```python
from build123d import *

# Parameters (mm, degrees)
BOSS_EXTRUDE1_DEPTH = 7.5
CUT_EXTRUDE3_DEPTH  = 5
SKETCH3_R           = 1.825
CUT_EXTRUDE4_DEPTH  = 13.5
SKETCH4_W           = 33.2
SKETCH4_H           = 26
CUT_EXTRUDE5_DEPTH  = 1
SKETCH5_W           = 2.5
SKETCH5_H           = 8
CUT_EXTRUDE6_DEPTH  = 5
BOSS_EXTRUDE2_DEPTH = 1
CUT_EXTRUDE8_DEPTH  = 10
SKETCH9_W           = 0.917517868
SKETCH9_H           = 1.289779541
SKETCH9_W_2         = 0.704402717
CUT_EXTRUDE9_DEPTH  = 1
CHAMFER1_SIZE       = 1
FILLET1_R           = 3.65


with BuildPart() as part:
    # Sketch1 → Boss-Extrude1 (new body)
    with BuildSketch(Plane(origin=(0, 0, 0), x_dir=(1, 0, 0), z_dir=(0, 1, 0))):
        with BuildLine():
            Line((-17.1, -15.5), (17.1, -15.5))
            ThreePointArc((17.1, -15.5), (18.514213562, -14.914213562), (19.1, -13.5))
            Line((19.1, -13.5), (19.1, 13.5))
            ThreePointArc((19.1, 13.5), (18.514213562, 14.914213562), (17.1, 15.5))
            Line((17.1, 15.5), (-17.1, 15.5))
            ThreePointArc((-17.1, 15.5), (-18.514213562, 14.914213562), (-19.1, 13.5))
            Line((-19.1, 13.5), (-19.1, -13.5))
            ThreePointArc((-19.1, -13.5), (-18.514213562, -14.914213562), (-17.1, -15.5))
        make_face()
    extrude(amount=BOSS_EXTRUDE1_DEPTH)

    # Sketch2 → Cut-Extrude3 (cut)
    with BuildSketch(Plane(origin=(0, 7.5, 0), x_dir=(1, 0, 0), z_dir=(0, 1, 0))):
        Polygon((-16.6, 5.5), (-9.1, 5.5), (-9.1, 13), (9.1, 13), (9.1, 5.5), (16.6, 5.5), (16.6, -5.5), (9.1, -5.5), (9.1, -13), (-9.1, -13), (-9.1, -5.5), (-16.6, -5.5), align=None)
    extrude(amount=-CUT_EXTRUDE3_DEPTH, mode=Mode.SUBTRACT)

    # Sketch3 → Cut-Extrude4 (cut)
    with BuildSketch(Plane(origin=(0, 7.5, 0), x_dir=(1, 0, 0), z_dir=(0, 1, 0))):
        with Locations((-12.425, 8.675)):
            Circle(SKETCH3_R)
        with Locations((12.425, 8.675)):
            Circle(SKETCH3_R)
        with Locations((12.425, -8.675)):
            Circle(SKETCH3_R)
        with Locations((-12.425, -8.675)):
            Circle(SKETCH3_R)
    extrude(amount=-CUT_EXTRUDE4_DEPTH, mode=Mode.SUBTRACT)

    # Sketch4 → Cut-Extrude5 (cut)
    with BuildSketch(Plane(origin=(0, 7.5, 0), x_dir=(1, 0, 0), z_dir=(0, 1, 0))):
        Rectangle(SKETCH4_W, SKETCH4_H)
    extrude(amount=-CUT_EXTRUDE5_DEPTH, mode=Mode.SUBTRACT)

    # Sketch5 → Cut-Extrude6 (cut)
    with BuildSketch(Plane(origin=(0, 7.5, 0), x_dir=(1, 0, 0), z_dir=(0, 1, 0))):
        with Locations((-17.85, 1.5)):
            Rectangle(SKETCH5_W, SKETCH5_H)
        with Locations((17.85, 1.5)):
            Rectangle(SKETCH5_W, SKETCH5_H)
    extrude(amount=-CUT_EXTRUDE6_DEPTH, mode=Mode.SUBTRACT)

    # Sketch6 → Boss-Extrude2 (add)
    with BuildSketch(Plane(origin=(0, 7.5, 0), x_dir=(1, 0, 0), z_dir=(0, 1, 0))):
        with BuildLine():
            Line((-17.95, 5.5), (-19.1, 5.5))
            Line((-19.1, 5.5), (-19.1, 13.5))
            ThreePointArc((-19.1, 13.5), (-18.514213562, 14.914213562), (-17.1, 15.5))
            Line((-17.1, 15.5), (17.1, 15.5))
            ThreePointArc((17.1, 15.5), (18.514213562, 14.914213562), (19.1, 13.5))
            Line((19.1, 13.5), (19.1, 5.5))
            Line((19.1, 5.5), (17.95, 5.5))
            Line((17.95, 5.5), (17.95, 13.5))
            ThreePointArc((17.95, 13.5), (17.701040764, 14.101040764), (17.1, 14.35))
            Line((17.1, 14.35), (-17.1, 14.35))
            ThreePointArc((-17.1, 14.35), (-17.701040764, 14.101040764), (-17.95, 13.5))
            Line((-17.95, 13.5), (-17.95, 5.5))
        make_face()
        with BuildLine():
            Line((-17.95, -2.5), (-19.1, -2.5))
            Line((-19.1, -2.5), (-19.1, -13.5))
            ThreePointArc((-19.1, -13.5), (-18.514213562, -14.914213562), (-17.1, -15.5))
            Line((-17.1, -15.5), (17.1, -15.5))
            ThreePointArc((17.1, -15.5), (18.514213562, -14.914213562), (19.1, -13.5))
            Line((19.1, -13.5), (19.1, -2.5))
            Line((19.1, -2.5), (17.95, -2.5))
            Line((17.95, -2.5), (17.95, -13.5))
            ThreePointArc((17.95, -13.5), (17.701040764, -14.101040764), (17.1, -14.35))
            Line((17.1, -14.35), (-17.1, -14.35))
            ThreePointArc((-17.1, -14.35), (-17.701040764, -14.101040764), (-17.95, -13.5))
            Line((-17.95, -13.5), (-17.95, -2.5))
        make_face()
    extrude(amount=BOSS_EXTRUDE2_DEPTH)

    # Sketch7 → Cut-Extrude8 (cut)
    with BuildSketch(Plane.XY.offset(15.5)):
        with BuildLine():
            Line((-5.1, 9), (3.9, 9))
            ThreePointArc((3.9, 9), (5.4, 7.5), (3.9, 6))
            Line((3.9, 6), (-5.1, 6))
            ThreePointArc((-5.1, 6), (-6.6, 7.5), (-5.1, 9))
        make_face()
    extrude(amount=-CUT_EXTRUDE8_DEPTH, mode=Mode.SUBTRACT)

    # Sketch9 → Cut-Extrude9 (cut)
    with BuildSketch(Plane(origin=(0, 7.5, 0), x_dir=(1, 0, 0), z_dir=(0, 1, 0))):
        with Locations((-6.141241066, -14.994889771)):
            Rectangle(SKETCH9_W, SKETCH9_H)
        with Locations((5.047798642, -14.994889771)):
            Rectangle(SKETCH9_W_2, SKETCH9_H)
    extrude(amount=CUT_EXTRUDE9_DEPTH, mode=Mode.SUBTRACT)

    # Chamfer1
    chamfer1_edges = [part.edges().sort_by_distance(p)[0] for p in [
        (-19.1, 0, 0),
        (-18.514213562, 0, -14.914213562),
        (0, 0, -15.5),
        (18.514213562, 0, -14.914213562),
        (19.1, 0, 0),
        (18.514213562, 0, 14.914213562),
        (0, 0, 15.5),
        (-18.514213562, 0, 14.914213562),
    ]]
    chamfer(chamfer1_edges, length=CHAMFER1_SIZE)

    # Fillet1
    fillet1_edges = [part.edges().sort_by_distance(p)[0] for p in [
        (-9.1, 4.5, 5.5),
        (-9.1, 4.5, -5.5),
        (9.1, 4.5, -5.5),
        (9.1, 4.5, 5.5),
    ]]
    fillet(fillet1_edges, radius=FILLET1_R)


solid = part.part
```
Part model, mm, in its own coordinate system. A direction names the side the tool comes from. Round coordinates to 2 decimals unless told otherwise and drop trailing zeros. Loops run counter-clockwise (first coordinate to the right, second up) from the corner with the lowest first, then second, coordinate; pieces in that order, holes last.
Item 1: Drill centre lines: line 1 (Z direction, x = 14, y = 5.75); line 2 (Z direction, x = 5, y = 4); line 3 (Z direction, x = 9, y = 7.75). Where is each one in solid material? Low to high.
Item 2: Cut at A-A, the plane y = 4. State how many separate pieces and enclosed holes the cut face has, then the cut area to 3 significant figures.
Item 3: Cut at B-B, the plane x = -8. Give the cut face in (y, z), then the cut area to 3 significant figures.
Item 4: Drop flat-ended pins along their axis: P1, Ø8.5, axis at x = -13.5, z = -10, coming from the +Y side; P2, Ø2.5, axis at x = 1.5, z = -11, coming from the +Y side; P3, Ø1.1, axis at y = 8, z = 15, coming from the -X side. Give the stop position or say it passes through.
Item 5: Mould opens along X. For faces 3 (the face through (-18.066, 0.382, -14.488)), 4 (the face through (14.166, 3.296, -9.223)), 5 (the face through (15, 8.5, 15)) say: +X half, -X half, draft (parallel to the pull), parting line (faces both ways), or undercut.
Item 6: Cut at D-D, the plane x = 13.5. Give the cut face in (y, z).
Item 7: 3-axis set-ups, long thin cutter, end or side, ignore diameter. For faces 1 (the face through (-18.088, 0.382, 14.466)), 2 (the face through (-16.6, 7, -9)): which of +Z, -Z, +X, -X, +Y, -Y reach the whole face in a straight line?
Item 8: Cut at C-C, the plane z = -8. Give the cut face in (x, y), then the cut area to 3 significant figures.
A:
1. line 1: z = -15.5 to -9.6, -7.75 to -5.5, 5.5 to 7.75, 9.6 to 15.5
1. line 2: z = -15.5 to -13, 13 to 15.5
1. line 3: z = -15.5 to -14.35, 14.35 to 15.5
2. separate pieces: 2
2. enclosed holes: 4
2. area: 449 mm2
3. outline: (0, -14.5) - (1, -15.5) - (8.5, -15.5) - (8.5, -14.35) - (7.5, -14.35) - (7.5, -13) - (2.5, -13) - (2.5, 13) - (7.5, 13) - (7.5, 14.35) - (8.5, 14.35) - (8.5, 15.5) - (1, 15.5) - (0, 14.5) - close
3. area: 104 mm2
4. P1: stops at y = 7.5
4. P2: stops at y = 2.5
4. P3: stops at x = -18.86
5. face 3: -X half
5. face 4: undercut
5. face 5: draft
6. outline: (0, -14.5) - (1, -15.5) - (8.5, -15.5) - (8.5, -14.35) - (7.5, -14.35) - (7.5, -13) - (6.5, -13) - (6.5, -10.15) - (0, -10.15) - close; (0, -7.2) - (6.5, -7.2) - (6.5, -5.5) - (2.5, -5.5) - (2.5, 5.5) - (6.5, 5.5) - (6.5, 7.2) - (0, 7.2) - close; (0, 10.15) - (6.5, 10.15) - (6.5, 13) - (7.5, 13) - (7.5, 14.35) - (8.5, 14.35) - (8.5, 15.5) - (1, 15.5) - (0, 14.5) - close
7. face 1: +Z, -X, -Y
7. face 2: +Y
8. outline: (-19.1, 1) - (-18.1, 0) - (-14.12, 0) - (-14.12, 6.5) - (-16.6, 6.5) - (-16.6, 7.5) - (-17.95, 7.5) - (-17.95, 8.5) - (-19.1, 8.5) - close; (-10.73, 0) - (10.73, 0) - (10.73, 6.5) - (9.29, 6.5) - (9.29, 2.5) - (-9.29, 2.5) - (-9.29, 6.5) - (-10.73, 6.5) - close; (14.12, 0) - (18.1, 0) - (19.1, 1) - (19.1, 8.5) - (17.95, 8.5) - (17.95, 7.5) - (16.6, 7.5) - (16.6, 6.5) - (14.12, 6.5) - close
8. area: 136 mm2
